Part model, mm, in its own coordinate system. Face numbers are marked on the shaded views. Coordinates: 2 decimals unless noted, no trailing zeros. Order: outer loops, then holes, each group sorted by start corner. A loop starts at its lowest first (then second) coordinate and runs counter-clockwise, first axis right, second up.
1) Wall check: L1, parallel to X at y = 70, z = 36; L2, parallel to X at y = 16, z = -55.5; L3, parallel to Z at x = -82, y = 42. Give the ranges that are in metal, low to high.
2) Pin check, flat tips, straight feed: pin 1 Ø2 at (y, z) = (60, -70.5) entering from -X; pin 2 Ø5 at (y, z) = (39, -8.5) entering from +X; pin 3 Ø3.5 at (x, y) = (38.5, 27.5) entering from -Z. Stop position of each tip, or through.
3) Cut at A-A (y = 9.5). List the corners of the cut face in (x, z), and give its area (3 significant figures).
4) Cut at C-C (z = 0). List the corners of the cut face in (x, y), and give its area (3 significant figures).
5) Mould opens along X. For the marked faces 1 and 2 say: +X half, -X half, draft (parallel to the pull), parting line (faces both ways), or undercut.
6) Cut at B-B (x = -19). List the corners of the cut face in (y, z), and give its area (3 significant figures).
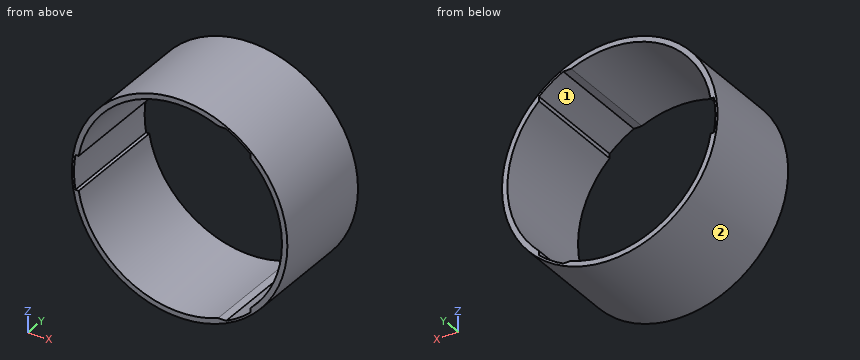
```python
from build123d import *

# Parameters (mm, degrees)
SKETCH1_R           = 100
SKETCH1_R_2         = 95
BOSS_EXTRUDE1_DEPTH = 100
CUT_EXTRUDE1_DEPTH  = 101


with BuildPart() as part:
    # Sketch1 → Boss-Extrude1 (new body)
    with BuildSketch(Plane(origin=(0, 0, 0), x_dir=(1, 0, 0), z_dir=(0, 1, 0))):
        Circle(SKETCH1_R)
        Circle(SKETCH1_R_2, mode=Mode.SUBTRACT)
    extrude(amount=BOSS_EXTRUDE1_DEPTH)

    # Sketch2 → Cut-Extrude1 (cut, through all)
    with BuildSketch(Plane(origin=(0, 100, 0), x_dir=(1, 0, 0), z_dir=(0, 1, 0))):
        with BuildLine():
            ThreePointArc((65.656830535, 72.754248014), (54.935999613, 81.154395731), (43.154094517, 87.98706795))
            Line((43.154094517, 87.98706795), (35.82284011, 87.98706795))
            ThreePointArc((35.82284011, 87.98706795), (51.651871532, 79.731324881), (65.656830535, 68.659890795))
            Line((65.656830535, 68.659890795), (65.656830535, 72.754248014))
        make_face()
        with BuildLine():
            ThreePointArc((43.154094517, -87.98706795), (54.935999613, -81.154395731), (65.656830535, -72.754248014))
            Line((65.656830535, -72.754248014), (65.656830535, -68.659890795))
            ThreePointArc((65.656830535, -68.659890795), (51.651871532, -79.731324881), (35.82284011, -87.98706795))
            Line((35.82284011, -87.98706795), (43.154094517, -87.98706795))
        make_face()
        with BuildLine():
            Line((-93.642938869, 16), (-96.685055722, 16))
            ThreePointArc((-96.685055722, 16), (-98, 0), (-96.685055722, -16))
            Line((-96.685055722, -16), (-93.642938869, -16))
            ThreePointArc((-93.642938869, -16), (-95, 0), (-93.642938869, 16))
        make_face()
    extrude(amount=-CUT_EXTRUDE1_DEPTH, mode=Mode.SUBTRACT)


solid = part.part
```
Geometry check:
1. L1: x = -93.3 to -87.91, 87.91 to 93.3
1. L2: x = -83.19 to -77.1, 77.1 to 83.19
1. L3: z = -57.24 to -47.97, 47.97 to 57.24
2. pin 1: stops at x = -71.9
2. pin 2: stops at x = 99.82
2. pin 3: stops at z = -93
3. outline: circle Ø200 at (0, 0); hole (-96.69, -16) - (-93.64, -16) arc R95 ccw to (35.82, -87.99) - (43.15, -87.99) arc R98 ccw to (65.66, -72.75) - (65.66, -68.66) arc R95 ccw to (65.66, 68.66) - (65.66, 72.75) arc R98 ccw to (43.15, 87.99) - (35.82, 87.99) arc R95 ccw to (-93.64, 16) - (-96.69, 16) arc R98 ccw to start
3. area: 2,780 mm2
4. outline: (-100, 0) - (-98, 0) - (-98, 100) - (-100, 100) - close; (95, 0) - (100, 0) - (100, 100) - (95, 100) - close
4. area: 700 mm2
5. face 1: undercut
5. face 2: parting line
6. outline: (0, -98.18) - (100, -98.18) - (100, -93.08) - (0, -93.08) - close; (0, 93.08) - (100, 93.08) - (100, 98.18) - (0, 98.18) - close
6. area: 1,020 mm2
